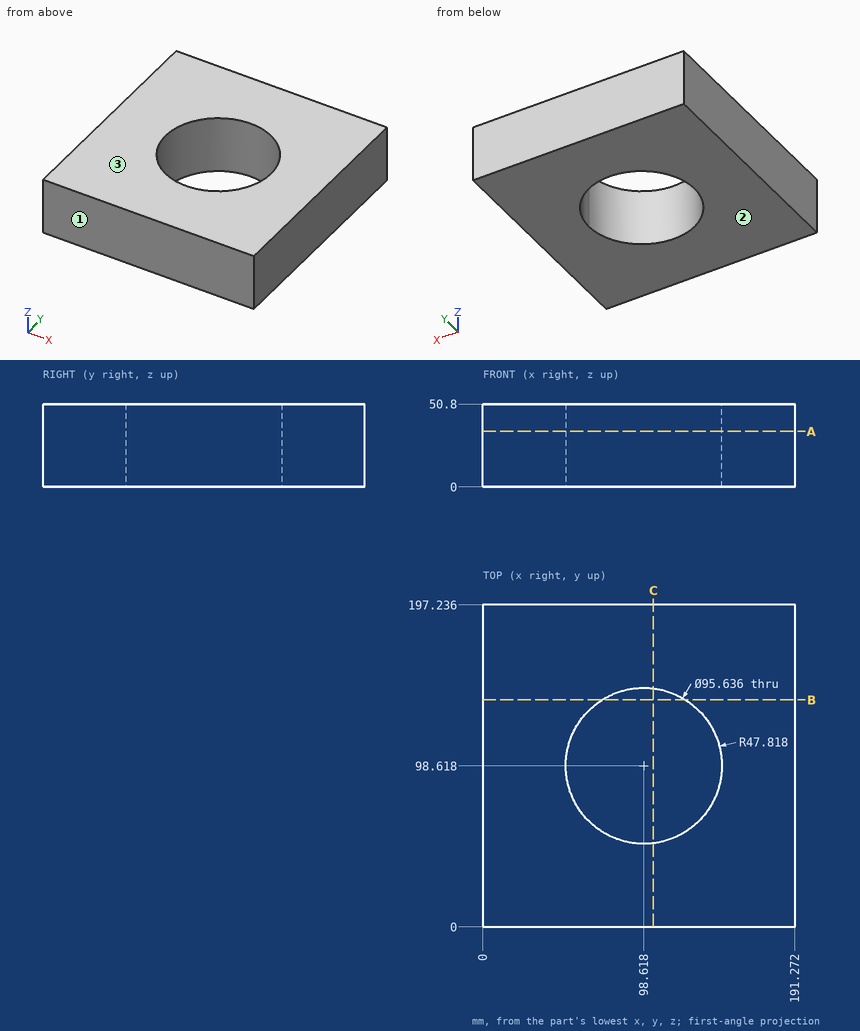
Verification items for this drawing (mm, ordinates from the low corner). Coordinates: 2 decimals unless noted, no trailing zeros. Loops run counter-clockwise (first coordinate to the right, second up) from the corner with the lowest first, then second, coordinate; pieces in that order, holes last.
Item 1: Thickness scan on line 1 (X direction, y = 78, z = 17); line 2 (X direction, y = 114, z = 15.5) (1 decimal); line 3 (Y direction, x = 69, z = 34.5). Record the ranges inside material, lowest first.
Item 2: Sectioned sample at B-B, the plane y = 139. Record the boundary of the cut face in (x, z).
Item 3: Release check for a two-part mould opening along Z. For the marked faces 1, 2 and 3 record: released by +Z, released by -Z, zero draft, split by the parting line, or undercut.
Item 4: Sectioned sample at C-C, the plane x = 104.5. Record the boundary of the cut face in (y, z), then the cut area to 3 significant figures.
Item 5: Sectioned sample at A-A, the plane z = 34. Record the boundary of the cut face in (x, y), then the cut area to 3 significant figures.
Check result:
1. line 1: x = 0 to 55.47, 141.76 to 191.27
1. line 2: x = 0 to 53.3, 143.9 to 191.3
1. line 3: y = 0 to 61.08, 136.16 to 197.24
2. outline: (0, 0) - (73.01, 0) - (73.01, 50.8) - (0, 50.8) - close; (124.23, 0) - (191.27, 0) - (191.27, 50.8) - (124.23, 50.8) - close
3. face 1: zero draft
3. face 2: released by -Z
3. face 3: released by +Z
4. outline: (0, 0) - (51.16, 0) - (51.16, 50.8) - (0, 50.8) - close; (146.07, 0) - (197.24, 0) - (197.24, 50.8) - (146.07, 50.8) - close
4. area: 5,200 mm2
5. outline: (0, 0) - (191.27, 0) - (191.27, 197.24) - (0, 197.24) - close; hole circle Ø95.64 at (98.62, 98.62)
5. area: 30,500 mm2
